Geometry: final body of the model. Coordinates: model frame, mm. Face numbers are marked on the shaded views. A direction names the side the tool comes from. Give positions to 0.01 mm unless a question says otherwise; leave off trailing zeros. Write each loop counter-clockwise with the first axis right and the second up, starting at its lowest first coordinate (ties: lowest second). Pieces come first, ordered by that corner, then holes.
Q1. Section B-B (y = 29). Return the cut outline in (x, z).
Q2. Reachability of the marked faces 1, 2 and 3 from +Z, -Z, +X, -X, +Y, -Y: full face, straight path, thin tool, end or side. Return the list, or none.
Q3. Line query: line 1 (Y direction, x = 0.65, z = -1.6); line 2 (X direction, y = 33, z = 1); line 3 (Z direction, x = 0.4, y = 33). Output: solid intervals per line, ascending.
Q4. Section A-A (z = -1.1). Return the cut outline in (x, y), plus the area to 3 significant figures.
Q5. Section C-C (x = 0). Return the cut outline in (y, z).
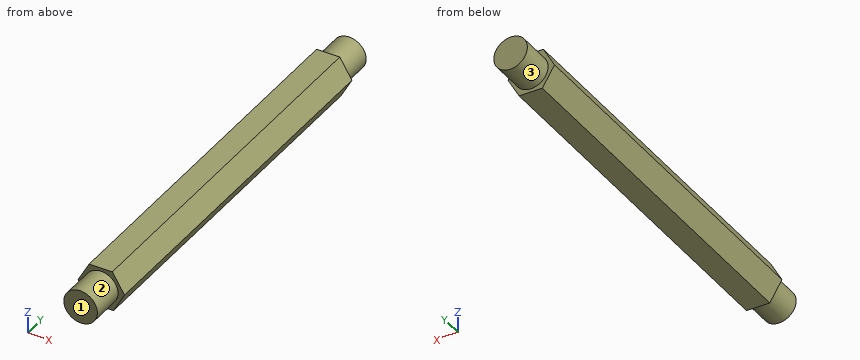
from build123d import *

# Parameters (mm, degrees)
SKETCH1_R           = 1.5
BOSS_EXTRUDE1_DEPTH = 3
BOSS_EXTRUDE2_DEPTH = 33
SKETCH3_R           = 1.5
BOSS_EXTRUDE3_DEPTH = 3


with BuildPart() as part:
    # Sketch1 → Boss-Extrude1 (new body)
    with BuildSketch(Plane(origin=(0, 0, 0), x_dir=(1, 0, 0), z_dir=(0, 1, 0))):
        with Locations(Location((0, 0, 0), (0, 0, 270))):
            Circle(SKETCH1_R)
    extrude(amount=BOSS_EXTRUDE1_DEPTH)

    # Sketch2 → Boss-Extrude2 (add)
    with BuildSketch(Plane(origin=(0, 3, 0), x_dir=(1, 0, 0), z_dir=(0, 1, 0))):
        Polygon((-0.98915483, 1.827996915), (-2.077669182, 0.057365247), (-1.088514352, -1.770631668), (0.98915483, -1.827996915), (2.077669182, -0.057365247), (1.088514352, 1.770631668), align=None)
    extrude(amount=BOSS_EXTRUDE2_DEPTH)

    # Sketch3 → Boss-Extrude3 (add)
    with BuildSketch(Plane(origin=(0, 36, 0), x_dir=(1, 0, 0), z_dir=(0, 1, 0))):
        with Locations(Location((0, 0, 0), (0, 0, 270))):
            Circle(SKETCH3_R)
    extrude(amount=BOSS_EXTRUDE3_DEPTH)


solid = part.part
Computed:
1. outline: (-2.08, -0.06) - (-0.99, -1.83) - (1.09, -1.77) - (2.08, 0.06) - (0.99, 1.83) - (-1.09, 1.77) - close
2. face 1: +Z, -Z, +X, -X, -Y
2. face 2: -Y
2. face 3: +Y
3. line 1: y = 3 to 36
3. line 2: x = -1.51 to 1.5
3. line 3: z = -1.79 to 1.81
4. outline: (-1.44, 3) - (-1.02, 3) - (-1.02, 0) - (1.02, 0) - (1.02, 3) - (1.45, 3) - (1.45, 36) - (1.02, 36) - (1.02, 39) - (-1.02, 39) - (-1.02, 36) - (-1.44, 36) - close
4. area: 108 mm2
5. outline: (0, -1.5) - (3, -1.5) - (3, -1.8) - (36, -1.8) - (36, -1.5) - (39, -1.5) - (39, 1.5) - (36, 1.5) - (36, 1.8) - (3, 1.8) - (3, 1.5) - (0, 1.5) - close
